from build123d import *

# Parameters (mm, degrees)
BOSS_EXTRUDE1_DEPTH      = 5.73
BOSS_EXTRUDE1_DEPTH_BACK = 5.73
BOSS_EXTRUDE2_DEPTH      = 11.46
BOSS_EXTRUDE3_DEPTH      = 11.46
BOSS_EXTRUDE4_DEPTH      = 2.999321
SKETCH7_R                = 3.54
CUT_EXTRUDE2_DEPTH       = 2.999322
BOSS_EXTRUDE5_DEPTH      = 3
SKETCH11_R               = 1.52
CUT_EXTRUDE3_DEPTH       = 3
BOSS_EXTRUDE6_DEPTH      = 3.000001
BOSS_EXTRUDE7_DEPTH      = 4.24753
SKETCH15_R               = 1.75
CUT_EXTRUDE4_DEPTH       = 4.24753


with BuildPart() as part:
    # Sketch1 → Boss-Extrude1 (new, two sides: drawn at the far end of the back side and taken through both)
    with BuildSketch(Plane.XY.offset(-BOSS_EXTRUDE1_DEPTH_BACK)):
        Polygon((32.166139185, 36.798009468), (35.166138746, 39.798007166), (38.166139237, 36.798004811), (38.166139237, 4.578006273), (35.166137814, 1.578006712), (32.166137322, 4.578009067), (35.166137814, 7.578007696), (35.166137814, 33.798008976), align=None)
    extrude(amount=BOSS_EXTRUDE1_DEPTH + BOSS_EXTRUDE1_DEPTH_BACK)

    # Sketch2 → Boss-Extrude2 (add)
    with BuildSketch(Plane.XY.offset(5.73)):
        Polygon((32.166139185, 36.798009468), (20.006139185, 36.798009468), (20.006139185, 39.797331447), (32.166139185, 39.797331447), (35.165463026, 39.797331447), align=None)
    extrude(amount=-BOSS_EXTRUDE2_DEPTH)

    # Sketch3 → Boss-Extrude3 (add)
    with BuildSketch(Plane.XY.offset(5.73)):
        Polygon((32.166137322, 4.578009067), (35.166137814, 1.578006712), (32.166137322, 1.578006712), (20.006137322, 1.578006712), (20.006137322, 4.578009067), align=None)
    extrude(amount=-BOSS_EXTRUDE3_DEPTH)

    # Sketch4 → Boss-Extrude4 (add)
    with BuildSketch(Plane(origin=(0, 39.797331447, 0), x_dir=(1, 0, 0), z_dir=(0, 1, 0))):
        with BuildLine():
            Line((20.006139185, 5.73), (20.006139185, -5.73))
            ThreePointArc((20.006139185, -5.73), (7.794878848, 0), (20.006139185, 5.73))
        make_face()
    extrude(amount=-BOSS_EXTRUDE4_DEPTH)

    # Sketch7 → Cut-Extrude2 (cut)
    with BuildSketch(Plane(origin=(0, 39.797331447, 0), x_dir=(1, 0, 0), z_dir=(0, 1, 0))):
        with Locations(Location((15.244878848, 0, 0), (0, 0, 270))):
            Circle(SKETCH7_R)
    extrude(amount=-CUT_EXTRUDE2_DEPTH, mode=Mode.SUBTRACT)

    # Sketch9 → Boss-Extrude5 (add)
    with BuildSketch(Plane(origin=(0, 1.578006712, 0), x_dir=(-1, 0, 0), z_dir=(0, -1, 0))):
        with BuildLine():
            Line((-20.006139185, -5.73), (-15.244878848, -5.73))
            ThreePointArc((-15.244878848, -5.73), (-9.514878848, 0), (-15.244878848, 5.73))
            Line((-15.244878848, 5.73), (-20.006137322, 5.73))
            Line((-20.006137322, 5.73), (-20.006139185, -5.73))
        make_face()
    extrude(amount=-BOSS_EXTRUDE5_DEPTH)

    # Sketch11 → Cut-Extrude3 (cut)
    with BuildSketch(Plane(origin=(0, 1.578006712, 0), x_dir=(-1, 0, 0), z_dir=(0, -1, 0))):
        with Locations(Location((-15.244878848, 0, 0), (0, 0, 90))):
            Circle(SKETCH11_R)
    extrude(amount=-CUT_EXTRUDE3_DEPTH, mode=Mode.SUBTRACT)

    # Sketch12 → Boss-Extrude6 (add)
    with BuildSketch(Plane(origin=(38.166139237, 0, 0), x_dir=(0, 0, -1), z_dir=(1, 0, 0))):
        Polygon((-5.73, 32.188009468), (-5.73, 9.188006273), (-15.106235919, 18.564242191), (-15.106235919, 22.811773549), align=None)
    extrude(amount=-BOSS_EXTRUDE6_DEPTH)

    # Sketch14 → Boss-Extrude7 (add)
    with BuildSketch(Plane(origin=(0, 18.564244712, 0), x_dir=(-1, 0, 0), z_dir=(0, -1, 0))):
        with BuildLine():
            Line((-38.166139237, -15.106235919), (-38.166139237, -17.856235919))
            Line((-38.166139237, -17.856235919), (-30.594801522, -23.440347499))
            ThreePointArc((-30.594801522, -23.440347499), (-28.233323063, -24.573172743), (-25.620768045, -24.758725505))
            Line((-25.620768045, -24.758725505), (-22.565521767, -24.398737054))
            ThreePointArc((-22.565521767, -24.398737054), (-21.460785016, -24.442412716), (-20.423400376, -24.824752827))
            ThreePointArc((-20.423400376, -24.824752827), (-13.74802539, -22.300713773), (-20.66830721, -20.556837667))
            ThreePointArc((-20.66830721, -20.556837667), (-21.746000534, -21.192615252), (-22.977558626, -21.413750285))
            Line((-22.977558626, -21.413750285), (-25.055666544, -21.413750285))
            ThreePointArc((-25.055666544, -21.413750285), (-27.436600146, -20.996390727), (-29.53361792, -19.794080338))
            Line((-29.53361792, -19.794080338), (-35.166137814, -15.106235919))
            Line((-35.166137814, -15.106235919), (-38.166139237, -15.106235919))
        make_face()
    extrude(amount=-BOSS_EXTRUDE7_DEPTH)

    # Sketch15 → Cut-Extrude4 (cut)
    with BuildSketch(Plane(origin=(0, 18.564244712, 0), x_dir=(-1, 0, 0), z_dir=(0, -1, 0))):
        with Locations(Location((-17.41764683, -22.48214533, 0), (0, 0, 90))):
            Circle(SKETCH15_R)
    extrude(amount=-CUT_EXTRUDE4_DEPTH, mode=Mode.SUBTRACT)


solid = part.part
Work out the finished part from the listing and answer in its coordinate system (mm). A direction names the side the tool comes from. Round coordinates to 2 decimals unless told otherwise and drop trailing zeros. Loops run counter-clockwise (first coordinate to the right, second up) from the corner with the lowest first, then second, coordinate; pieces in that order, holes last. Notation, with made-up numbers: (48.5, 82.5) - (91.5, 82.5) arc R18 cw to (91.5, 111.5) - close; hole circle Ø7 at (66.5, 61). An arc over 180 degrees is marked (long way). One line per item, written item: value.
Q1. For faces 1 (the cylindrical face through (27.4, 20.66, 21.01)), 2 (the flat face through (34.43, 20.66, 20.61)), 3 (the flat face through (26, 36.798, 0)), determine the directions among +Z, -Z, +X, -X, +Y, -Y from which every point of the face is accessible in a straight line to the end or side of a thin tool.
Check values:
face 1: -Z, +Y, -Y
face 2: +Z, +X, +Y, -Y
face 3: +Z, -Z, -X
Q2. Find section B-B on y = 22. Give the vertices of the cut face in (x, z).
Check values:
outline: (20.42, 24.82) arc R3.74 ccw (long way) to (20.67, 20.56) arc R3.54 cw to (22.98, 21.41) - (25.06, 21.41) arc R7 cw to (29.53, 19.79) - (35.17, 15.11) - (35.17, -5.73) - (38.17, -5.73) - (38.17, 17.86) - (30.59, 23.44) arc R7 ccw to (25.62, 24.76) - (22.57, 24.4) arc R3.54 cw to start; hole circle Ø3.5 at (17.42, 22.48)
Q3. Straight lines are drawn through the part: probe 1 along X at (y, z) = (29, -3); probe 2 along X at (y, z) = (2.5, 0); probe 3 along Y at (x, z) = (36, 15.5). For each, find the intervals that lie inside material, in ascending order.
Check values:
probe 1: 35.17 to 38.17
probe 2: 9.51 to 13.72, 16.76 to 36.09
probe 3: 18.56 to 22.81
Q4. The mould has two halves that part along X. Classify faces 4 (the flat face through (22, 1.578, 0)), 5 (the cylindrical face through (21.48, 20.66, 24.44)), 6 (the flat face through (35.166, 21, 0)): +X half, -X half, draft (parallel to the pull), parting line (faces both ways), or undercut.
Check values:
face 4: draft
face 5: undercut
face 6: -X half
Q5. Find section A-A on z = 0. State how many separate pieces and enclosed holes the cut face has, and give its area (3 significant figures).
Check values:
separate pieces: 3
enclosed holes: 0
area: 243 mm2
Q6. Each of these flat-tipped pins is pushed along its axis until it touches: pin 1 Ø3.5 at (x, z) = (15.24, 0) entering from +Y; pin 2 Ø12.5 at (x, z) = (25.5, 23.5) entering from -Y; pin 3 Ø1.5 at (x, y) = (14, 21.5) entering from +Z. Where does it stop, or does it pass through?
Check values:
pin 1: y = 4.58
pin 2: y = 18.56
pin 3: z = 25.07
Q7. Find section D-D on y = 29.5. Give the vertices of the cut face in (x, z).
Check values:
outline: (35.17, -5.73) - (38.17, -5.73) - (38.17, 8.42) - (35.17, 8.42) - close
